Check sheet for the modelled part. Datum: model origin and axes. Units: mm. A direction names the side the tool comes from. Round coordinates to 2 decimals unless told otherwise and drop trailing zeros. Order: outer loops, then holes, each group sorted by start corner. A loop starts at its lowest first (then second) coordinate and runs counter-clockwise, first axis right, second up. Notation, with made-up numbers: (-34, -15) -> (-7, -15) arc R34 ccw to (-7, 22) -> close; hole circle Ø5 at (38, -25.5). An arc over 180 degrees is marked (long way). Answer in a Markdown table with one row per item. Add a question column.
1. Access from +Z, -Z, +X, -X, +Y, -Y to the whole of each face (thin tool, end or side, straight path). Record for faces 1 (the flat face through (4.5, 394, 0)), 2 (the flat face through (23, 0, -45)).
2. Sectioned sample at B-B, the plane z = 0. Record the boundary of the cut face in (x, y).
3. Sectioned sample at A-A, the plane y = 154.5. Record the boundary of the cut face in (x, z).
4. Material ranges on L1, parallel to Z at x = 42.5, y = 309.5; L2, parallel to X at y = 750, z = -45.5; L3, parallel to X at y = 352, z = -10, recorded low to high. Write a range as from..to.
5. Depth check by flat-ended pin: P1, Ø10, axis at x = 26.44, y = 350, coming from the +Z side. Enter the tip coordinate at first touch or a pass-through.
6. Draft check along Y on faces 3 (the cylindrical face through (27.23, 756.05, -46.15)), 4 (the cylindrical face through (23.6, 344.6, 46.3)), 5 (the flat face through (27, 394, -42.4)), 6 (the flat face through (23, 0, 45)). Enter one of: +Y half, -Y half, draft (parallel to the pull), parting line (faces both ways), or undercut.
```python
from build123d import *

# Parameters (mm, degrees)
EXTRUDE_1_DEPTH          = 800
CUT_EXTRUDE_1_DEPTH      = 803.87981666
CUT_EXTRUDE_1_DEPTH_BACK = 803.87981666
FILLET_1_R               = 10
CUT_EXTRUDE_2_DEPTH      = 808.536996057
CUT_EXTRUDE_2_DEPTH_BACK = 808.536996057
SKETCH_3_R               = 6.1


with BuildPart() as part:
    # Эскиз1 → Бобышка-Вытянуть1 (new body)
    with BuildSketch(Plane(origin=(0, 0, 0), x_dir=(1, 0, 0), z_dir=(0, 1, 0))):
        with BuildLine():
            Line((0, -50), (0, 50))
            Line((0, 50), (46, 50))
            Line((46, 50), (46, 46.4))
            ThreePointArc((46, 46.4), (44.828427125, 43.571572875), (42, 42.4))
            Line((42, 42.4), (11.5, 42.4))
            ThreePointArc((11.5, 42.4), (6.550252532, 40.349747468), (4.5, 35.4))
            Line((4.5, 35.4), (4.5, -35.4))
            ThreePointArc((4.5, -35.4), (6.550252532, -40.349747468), (11.5, -42.4))
            Line((11.5, -42.4), (42, -42.4))
            ThreePointArc((42, -42.4), (44.828427125, -43.571572875), (46, -46.4))
            Line((46, -46.4), (46, -50))
            Line((46, -50), (0, -50))
        make_face()
    extrude(amount=EXTRUDE_1_DEPTH)

    # Эскиз2 → Вырез-Вытянуть1 (cut, two sides: drawn at the far end of the back side and taken through both)
    with BuildSketch(Plane.ZY.offset(-CUT_EXTRUDE_1_DEPTH_BACK)):
        with BuildLine():
            Line((-22.5, 35), (-22.5, 0))
            Line((-22.5, 0), (22.5, 0))
            Line((22.5, 0), (22.5, 35))
            ThreePointArc((22.5, 35), (0, 57.5), (-22.5, 35))
        make_face()
    extrude(amount=CUT_EXTRUDE_1_DEPTH + CUT_EXTRUDE_1_DEPTH_BACK, mode=Mode.SUBTRACT)

    # Скругление1
    fillet_1_edges = [part.edges().sort_by_distance(p)[0] for p in [
        (2.25, 0, -22.5),
        (2.25, 0, 22.5),
    ]]
    fillet(fillet_1_edges, radius=FILLET_1_R)

    # Эскиз3 → Вырез-Вытянуть2 (cut, two sides: drawn at the far end of the back side and taken through both)
    with BuildSketch(Plane(origin=(0, 0, -50), x_dir=(-1, 0, 0), z_dir=(0, 0, -1)).offset(-CUT_EXTRUDE_2_DEPTH_BACK)):
        with Locations((-26.44, 750)):
            Circle(SKETCH_3_R)
        with Locations((-26.44, 650)):
            Circle(SKETCH_3_R)
        with Locations((-26.44, 550)):
            Circle(SKETCH_3_R)
        with Locations((-26.44, 450)):
            Circle(SKETCH_3_R)
        with Locations((-26.44, 350)):
            Circle(SKETCH_3_R)
        with Locations((-26.44, 250)):
            Circle(SKETCH_3_R)
    extrude(amount=CUT_EXTRUDE_2_DEPTH + CUT_EXTRUDE_2_DEPTH_BACK, mode=Mode.SUBTRACT)


solid = part.part
```
Answer key:
| question | item | result |
|---|---|---|
| 1 | face 1 | +X, +Y, -Y |
| 1 | face 2 | +Z, -Z, +X, -X, -Y |
| 2 | outline | (0, 57.5) -> (4.5, 57.5) -> (4.5, 800) -> (0, 800) -> close |
| 3 | outline | (0, -50) -> (46, -50) -> (46, -46.4) arc R4 ccw to (42, -42.4) -> (11.5, -42.4) arc R7 cw to (4.5, -35.4) -> (4.5, 35.4) arc R7 cw to (11.5, 42.4) -> (42, 42.4) arc R4 ccw to (46, 46.4) -> (46, 50) -> (0, 50) -> close |
| 4 | L1 | z = -50..-42.43, 42.43..50 |
| 4 | L2 | x = 0..20.34, 32.54..45.9 |
| 4 | L3 | x = 0..4.5 |
| 5 | P1 | passes through |
| 6 | face 3 | undercut |
| 6 | face 4 | undercut |
| 6 | face 5 | draft |
| 6 | face 6 | -Y half |
